Verification items for this drawing (mm, ordinates from the low corner). Round coordinates to 2 decimals unless told otherwise and drop trailing zeros. Write each loop counter-clockwise with the first axis right and the second up, starting at its lowest first coordinate (ties: lowest second). Pieces come first, ordered by that corner, then holes. Notation, with made-up numbers: (-13.5, -31) -> (30.5, -31) arc R21 cw to (30.5, -22) -> close; hole circle Ø10 at (61, 5). An arc over 180 degrees is marked (long way). One line per item, written item: value.
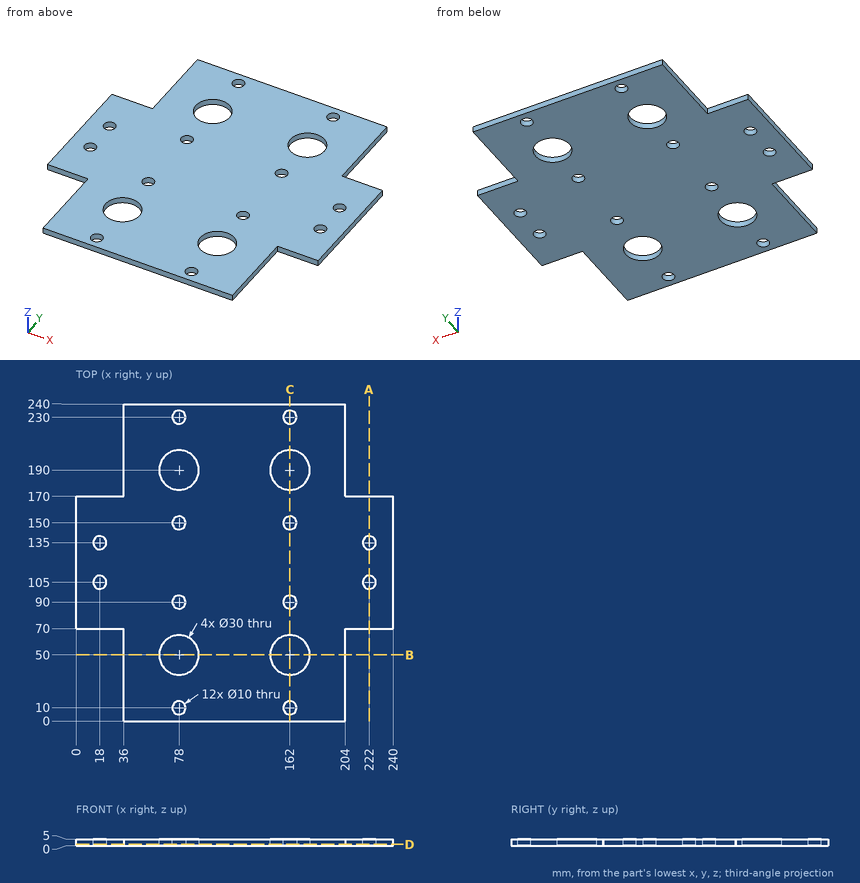
Item 1: Material ranges on line 1 along Y through (x, z) = (18, 1.85); line 2 along X through (y, z) = (190.5, 4.55); line 3 along X through (y, z) = (230.5, 4), recorded low to high.
Result set:
line 1: 70 to 100, 110 to 130, 140 to 170
line 2: 36 to 63.01, 92.99 to 147.01, 176.99 to 204
line 3: 36 to 73.03, 82.97 to 157.03, 166.97 to 204
Item 2: Sectioned sample at D-D (z = 0.9). State how many separate pieces and enclosed holes the cut face has, then the cut area to 4 significant figures.
Result set:
separate pieces: 1
enclosed holes: 16
area: 43,750 mm^2
Item 3: Depth check by flat-ended pin: pin 1 (2.5 mm diameter, centred on y = 50, z = 2.5, fed in from +X); pin 2 (2.5 mm diameter, centred on x = 25.5, z = 3.5, fed in from -Y); pin 3 (1.5 mm diameter, centred on y = 201, z = 2, fed in from -X). Enter the tip coordinate at first touch or a pass-through.
Result set:
pin 1: x = 204
pin 2: y = 70
pin 3: x = 36
Item 4: Sectioned sample at C-C (x = 162). Enter the section's corners in (y, z).
Result set:
outline: (0, 0) -> (5, 0) -> (5, 5) -> (0, 5) -> close; (15, 0) -> (35, 0) -> (35, 5) -> (15, 5) -> close; (65, 0) -> (85, 0) -> (85, 5) -> (65, 5) -> close; (95, 0) -> (145, 0) -> (145, 5) -> (95, 5) -> close; (155, 0) -> (175, 0) -> (175, 5) -> (155, 5) -> close; (205, 0) -> (225, 0) -> (225, 5) -> (205, 5) -> close; (235, 0) -> (240, 0) -> (240, 5) -> (235, 5) -> close
Item 5: Sectioned sample at A-A (x = 222). Enter the section's corners in (y, z), then the cut area to 3 significant figures.
Result set:
outline: (70, 0) -> (100, 0) -> (100, 5) -> (70, 5) -> close; (110, 0) -> (130, 0) -> (130, 5) -> (110, 5) -> close; (140, 0) -> (170, 0) -> (170, 5) -> (140, 5) -> close
area: 400 mm^2
Item 6: Sectioned sample at B-B (y = 50). Enter the section's corners in (x, z).
Result set:
outline: (36, 0) -> (63, 0) -> (63, 5) -> (36, 5) -> close; (93, 0) -> (147, 0) -> (147, 5) -> (93, 5) -> close; (177, 0) -> (204, 0) -> (204, 5) -> (177, 5) -> close
